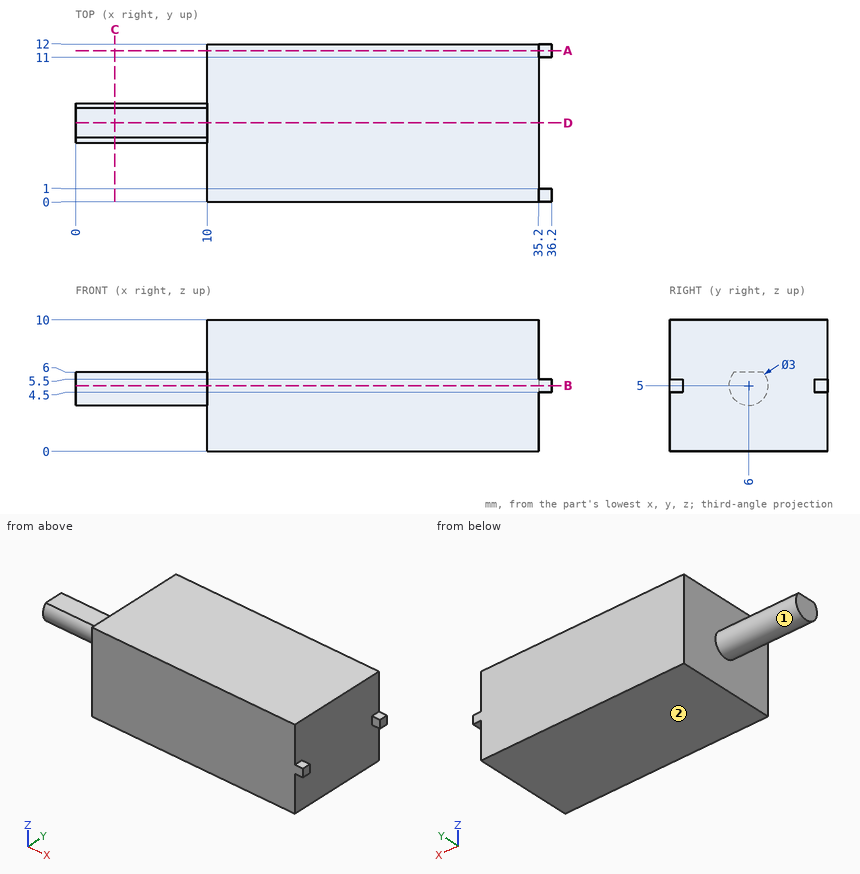
Input: dimensioned drawing with shaded views. Units: mm. Origin: part minimum x, y, z. A direction names the side the tool comes from. Give positions to 0.01 mm unless a question says otherwise; leave off trailing zeros. Order: outer loops, then holes, each group sorted by start corner. A loop starts at its lowest first (then second) coordinate and runs counter-clockwise, first axis right, second up. Notation, with made-up numbers: (21, 62) -> (25, 62) arc R15 cw to (25, 77) -> close; hole circle Ø11 at (37, 58). An arc over 180 degrees is marked (long way). Write item = value, one per line.
Item 1: Contact query for flat-ended pins moving along their axis: pin 1 (6 mm diameter, centred on y = 7.5, z = 8.5, fed in from -X); pin 2 (3 mm diameter, centred on y = 5.5, z = 7, fed in from +X); pin 3 (0.8 mm diameter, centred on x = 36, y = 0.5, fed in from -Z); pin 4 (2.5 mm diameter, centred on x = 3, y = 6, fed in from +Z). Output: stop coordinate, or through.
Check result:
pin_1 = 0
pin_2 = 35.2
pin_3 = 4.5
pin_4 = 6
Item 2: Section query A-A (y = 11.5). Output: boundary loops of the cut face in (x, z).
Check result:
outline = (10, 0) -> (35.2, 0) -> (35.2, 4.5) -> (36.2, 4.5) -> (36.2, 5.5) -> (35.2, 5.5) -> (35.2, 10) -> (10, 10) -> close
Item 3: Set-up query: the marked faces 1 and 2. Return all of +Z, -Z, +X, -X, +Y, -Y with unobstructed straight access to the full face (end or side cutting, diameter ignored); none if empty.
Check result:
face_1 = -X
face_2 = -Z, +X, -X, +Y, -Y
Item 4: Section query D-D (y = 6). Output: boundary loops of the cut face in (x, z), then the cut area to 3 significant figures.
Check result:
outline = (0, 3.5) -> (10, 3.5) -> (10, 0) -> (35.2, 0) -> (35.2, 10) -> (10, 10) -> (10, 6) -> (0, 6) -> close
area = 277 mm²
Item 5: Section query B-B (z = 5). Output: boundary loops of the cut face in (x, y).
Check result:
outline = (0, 4.5) -> (10, 4.5) -> (10, 0) -> (36.2, 0) -> (36.2, 1) -> (35.2, 1) -> (35.2, 11) -> (36.2, 11) -> (36.2, 12) -> (10, 12) -> (10, 7.5) -> (0, 7.5) -> close
Item 6: Ray query, probe 1 along X at (y, z) = (6, 3.25); probe 2 along X at (y, z) = (6.25, 5.75); probe 3 along Y at (x, z) = (6, 5). Return the intervals inside material, ascending.
Check result:
probe_1 = 10 to 35.2
probe_2 = 0 to 35.2
probe_3 = 4.5 to 7.5
Item 7: Section query C-C (x = 3). Output: boundary loops of the cut face in (y, z).
Check result:
outline = (4.88, 6) arc R1.5 ccw (long way) to (7.12, 6) -> close
